Build history of the part. All positions in model axes, mm. A direction names the side the tool comes from. Give positions to 0.01 mm unless a question says otherwise; leave off trailing zeros. Write each loop counter-clockwise with the first axis right and the second up, starting at its lowest first coordinate (ties: lowest second). Pieces come first, ordered by that corner, then holes.
from build123d import *

# Parameters (mm, degrees)
SKETCH_2_W          = 110
SKETCH_2_H          = 108.5
EXTRUDE_1_DEPTH     = 10
CUT_EXTRUDE_1_DEPTH = 124.057151357
SKETCH_4_W          = 25
SKETCH_4_H          = 88.5
CUT_EXTRUDE_2_DEPTH = 78.897769544
CUT_EXTRUDE_3_DEPTH = 2
SKETCH_6_W          = 76
SKETCH_6_H          = 80
CUT_EXTRUDE_4_DEPTH = 78.666353719
CUT_EXTRUDE_5_DEPTH = 3
SKETCH_8_R          = 0.85
SKETCH_8_R_2        = 1.75
CUT_EXTRUDE_6_DEPTH = 78.666353719
SKETCH_9_R          = 1.75
CUT_EXTRUDE_7_DEPTH = 78.897769544


with BuildPart() as part:
    # 스케치2 → 보스-돌출1 (new body)
    with BuildSketch(Plane(origin=(0, 0, 0), x_dir=(1, 0, 0), z_dir=(0, 1, 0))):
        Rectangle(SKETCH_2_W, SKETCH_2_H)
    extrude(amount=EXTRUDE_1_DEPTH)

    # 스케치3 → 컷-돌출1 (cut, through all)
    with BuildSketch(Plane.ZY.offset(55)):
        Polygon((-54.25, 6.15), (-47.351234773, 6.104845063), (-48.25, 0), (-54.25, 0), align=None)
    extrude(amount=-CUT_EXTRUDE_1_DEPTH, mode=Mode.SUBTRACT)

    # 스케치4 → 컷-돌출2 (cut, through all)
    with BuildSketch(Plane(origin=(0, 10, 0), x_dir=(1, 0, 0), z_dir=(0, 1, 0))):
        with Locations((-42.5, -10)):
            Rectangle(SKETCH_4_W, SKETCH_4_H)
    extrude(amount=-CUT_EXTRUDE_2_DEPTH, mode=Mode.SUBTRACT)

    # 스케치5 → 컷-돌출3 (cut)
    with BuildSketch(Plane(origin=(0, 10, 0), x_dir=(1, 0, 0), z_dir=(0, 1, 0))):
        Polygon((52, -54.25), (-27, -54.25), (-27, 34.25), (-55, 34.25), (-55, 43.25), (52, 43.25), align=None)
    extrude(amount=-CUT_EXTRUDE_3_DEPTH, mode=Mode.SUBTRACT)

    # 스케치6 → 컷-돌출4 (cut, through all)
    with BuildSketch(Plane(origin=(0, 8, 0), x_dir=(1, 0, 0), z_dir=(0, 1, 0))):
        with Locations((12.5, -3.75)):
            Rectangle(SKETCH_6_W, SKETCH_6_H)
    extrude(amount=-CUT_EXTRUDE_4_DEPTH, mode=Mode.SUBTRACT)

    # 스케치7 → 컷-돌출5 (cut)
    with BuildSketch(Plane(origin=(0, 8, 0), x_dir=(1, 0, 0), z_dir=(0, 1, 0))):
        with BuildLine():
            Line((52, -54.25), (38, -54.25))
            Line((38, -54.25), (38, -50.25))
            Line((38, -50.25), (-7.5, -50.25))
            Line((-7.5, -50.25), (-7.5, -46.75))
            ThreePointArc((-7.5, -46.75), (-10, -44.25), (-12.5, -46.75))
            Line((-12.5, -46.75), (-12.5, -54.25))
            Line((-12.5, -54.25), (-25.5, -54.25))
            Line((-25.5, -54.25), (-25.5, 34.25))
            Line((-25.5, 34.25), (-55, 34.25))
            Line((-55, 34.25), (-55, 43.25))
            Line((-55, 43.25), (-12.5, 43.25))
            Line((-12.5, 43.25), (-12.5, 39.25))
            ThreePointArc((-12.5, 39.25), (-10, 36.75), (-7.5, 39.25))
            Line((-7.5, 39.25), (-7.5, 43.25))
            Line((-7.5, 43.25), (45.5, 43.25))
            Line((45.5, 43.25), (45.5, 39.25))
            ThreePointArc((45.5, 39.25), (46.232233047, 37.482233047), (48, 36.75))
            Line((48, 36.75), (50.5, 36.75))
            Line((50.5, 36.75), (50.5, -44.25))
            Line((50.5, -44.25), (48, -44.25))
            ThreePointArc((48, -44.25), (45.5, -46.75), (48, -49.25))
            Line((48, -49.25), (52, -49.25))
            Line((52, -49.25), (52, -54.25))
        make_face()
    extrude(amount=-CUT_EXTRUDE_5_DEPTH, mode=Mode.SUBTRACT)

    # 스케치8 → 컷-돌출6 (cut, through all)
    with BuildSketch(Plane(origin=(0, 8, 0), x_dir=(1, 0, 0), z_dir=(0, 1, 0))):
        with Locations(Location((-10, 39.25, 0), (0, 0, 270))):
            Circle(SKETCH_8_R)
        with Locations(Location((48, 39.25, 0), (0, 0, 270))):
            Circle(SKETCH_8_R)
        with Locations(Location((-10, -46.75, 0), (0, 0, 270))):
            Circle(SKETCH_8_R)
        with Locations(Location((48, -46.75, 0), (0, 0, 270))):
            Circle(SKETCH_8_R)
        with Locations(Location((-50, 38.75, 0), (0, 0, 270))):
            Circle(SKETCH_8_R_2)
        with Locations(Location((30.5, 39.75, 0), (0, 0, 270))):
            Circle(SKETCH_8_R_2)
        with Locations(Location((42, -51.75, 0), (0, 0, 270))):
            Circle(SKETCH_8_R_2)
        with Locations(Location((-20.5, -49.25, 0), (0, 0, 270))):
            Circle(SKETCH_8_R_2)
    extrude(amount=-CUT_EXTRUDE_6_DEPTH, mode=Mode.SUBTRACT)

    # 스케치9 → 컷-돌출7 (cut, through all)
    with BuildSketch(Plane(origin=(0, 10, 0), x_dir=(1, 0, 0), z_dir=(0, 1, 0))):
        with Locations(Location((-50, 50.75, 0), (0, 0, 270))):
            Circle(SKETCH_9_R)
        with Locations(Location((0, 50.75, 0), (0, 0, 270))):
            Circle(SKETCH_9_R)
        with Locations(Location((50, 50.75, 0), (0, 0, 270))):
            Circle(SKETCH_9_R)
    extrude(amount=-CUT_EXTRUDE_7_DEPTH, mode=Mode.SUBTRACT)


solid = part.part
(1) 3-axis set-ups, long thin cutter, end or side, ignore diameter. For faces 4 (the face through (-30, 5, 11)), 5 (the face through (51, 8, -7)), 6 (the face through (49, 7, -36.75)), 7 (the face through (-7.5, 7, -41)): which of +Z, -Z, +X, -X, +Y, -Y reach the whole face in a straight line?
(2) Drop flat-ended pins along their axis: pin 1 (0.9 mm diameter, centred on y = 6.5, z = -40.5, fed in from -X); pin 2 (1.5 mm diameter, centred on y = 2.5, z = -28.5, fed in from -X); pin 3 (4 mm diameter, centred on x = 16, z = -37, fed in from +Y). Give the stop position or say it passes through.
(3) Saw through at B-B, the plane z = -25.5. List the corners of the cut face in (x, y).
(4) Saw through at D-D, the plane y = 1.5. Give the number of separate pieces and of enclosed holes in the cut face, plus the area to 3 significant figures.
(5) Saw through at C-C, the plane x = -20.5. List the corners of the cut face in (y, z).
(6) Probe line 1 (X direction, y = 6, z = 46.75); line 2 (X direction, y = 8.25, z = -50.75); line 3 (X direction, y = 8.5, z = -21). List the from-to ranges inside material, lowest first.
(7) Mould opens along Z. For faces 1 (the face through (-43, 3, -34.25)), 2 (the face through (38, 7, 52)), 3 (the face through (-0.67, 8.085, -49.133)) say: +Z half, -Z half, draft (parallel to the pull), parting line (faces both ways), or undercut.
(8) Saw through at A-A, the plane x = 10. List the corners of the cut face in (y, z), plus the area to 3 significant figures.
Computed values:
1. face 4: +Z, -X, +Y, -Y
1. face 5: +Z, +Y
1. face 6: -X, +Y
1. face 7: +Y
2. pin 1: stops at x = -12.5
2. pin 2: stops at x = -30
2. pin 3: stops at y = 5
3. outline: (-30, 0) - (-25.5, 0) - (-25.5, 8) - (-27, 8) - (-27, 10) - (-30, 10) - close; (50.5, 0) - (55, 0) - (55, 10) - (52, 10) - (52, 8) - (50.5, 8) - close
4. separate pieces: 1
4. enclosed holes: 9
4. area: 2,910 mm2
5. outline: (0, -48.25) - (6.1, -47.35) - (6.15, -54.25) - (10, -54.25) - (10, -43.25) - (5, -43.25) - (5, -36.25) - (0, -36.25) - close; (0, 43.75) - (5, 43.75) - (5, 47.5) - (0, 47.5) - close; (0, 51) - (5, 51) - (5, 54.25) - (0, 54.25) - close
6. line 1: x = -30 to -25.5, -12.5 to -10.85, -9.15 to -7.5, 45.5 to 47.15, 48.85 to 55
6. line 2: x = -55 to -51.75, -48.25 to -1.75, 1.75 to 48.25, 51.75 to 55
6. line 3: x = -30 to -27, 52 to 55
7. face 1: +Z half
7. face 2: draft
7. face 3: undercut
8. outline: (0, -48.25) - (6.1, -47.35) - (6.15, -54.25) - (10, -54.25) - (10, -43.25) - (5, -43.25) - (5, -36.25) - (0, -36.25) - close; (0, 43.75) - (5, 43.75) - (5, 50.25) - (8, 50.25) - (8, 54.25) - (0, 54.25) - close
8. area: 170 mm2
